For this review, take the finished solid that the model builds, in its own axes (mm). Face numbers are marked on the shaded views. A direction names the side the tool comes from. Coordinates: 2 decimals unless noted, no trailing zeros. Loops run counter-clockwise (first coordinate to the right, second up) from the corner with the lowest first, then second, coordinate; pieces in that order, holes last. Notation, with made-up numbers: M -19,-10 L -9,-10 A7 ccw -9,-1 Z; hole C -13,78.5 d4. An arc over 180 degrees is marked long. Put each result on its own line as item: value.
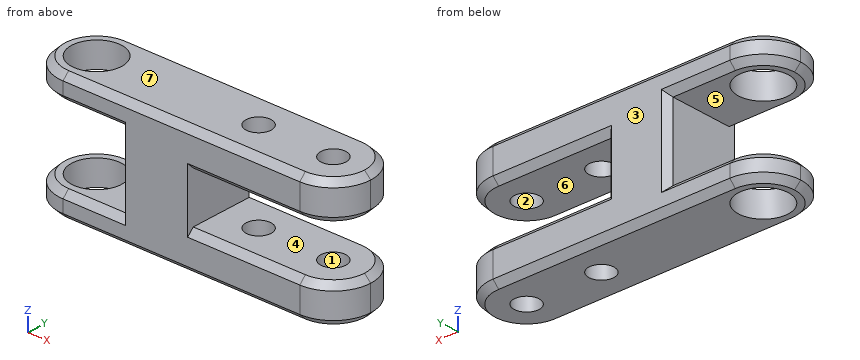
```python
from build123d import *

# Parameters (mm, degrees)
BOSS_EXTRUDE1_DEPTH       = 6
FILLET1_R                 = 3
F_4_0MM_DOWEL_HOLE1_D     = 4
F_4_0MM_DOWEL_HOLE1_DEPTH = 10
F_4_0MM_DOWEL_HOLE1_TIP   = 1.201721238
F_2_0MM_DOWEL_HOLE1_D     = 2
F_2_0MM_DOWEL_HOLE1_DEPTH = 10
F_2_0MM_DOWEL_HOLE1_TIP   = 0.600860619
CHAMFER1_SIZE             = 0.5


with BuildPart() as part:
    # Sketch2 → Boss-Extrude1 (new body)
    with BuildSketch(Plane(origin=(0, 0, 0), x_dir=(1, 0, 0), z_dir=(0, 1, 0))):
        Polygon((0, 3), (0, 5), (25, 5), (25, 2), (13, 2), (13, -2), (25, -2), (25, -5), (0, -5), (0, -3), (8, -3), (8, 3), align=None)
    extrude(amount=BOSS_EXTRUDE1_DEPTH)

    # Fillet1
    fillet1_edges = [part.edges().sort_by_distance(p)[0] for p in [
        (25, 6, -3.5),
        (25, 0, -3.5),
        (25, 0, 3.5),
        (25, 6, 3.5),
        (0, 6, 4),
        (0, 0, 4),
        (0, 0, -4),
        (0, 6, -4),
    ]]
    fillet(fillet1_edges, radius=FILLET1_R - 0.0001)  # a hair under: the kernel refuses the full size

    # Ø4.0mm Dowel Hole1
    with Locations(Plane.XY.offset(5)):
        with Locations((3, 3)):
            Hole(F_4_0MM_DOWEL_HOLE1_D / 2, depth=F_4_0MM_DOWEL_HOLE1_DEPTH)
            with Locations((0, 0, -(F_4_0MM_DOWEL_HOLE1_DEPTH + F_4_0MM_DOWEL_HOLE1_TIP / 2))):  # 118° drill point
                Cone(0, F_4_0MM_DOWEL_HOLE1_D / 2, F_4_0MM_DOWEL_HOLE1_TIP, mode=Mode.SUBTRACT)

    # Ø2.0mm Dowel Hole1
    with Locations(Plane(origin=(16, 3, 5), x_dir=(1, 0, 0), z_dir=(0, 0, 1))):
        with Locations((0, 0), (6, 0)):
            Hole(F_2_0MM_DOWEL_HOLE1_D / 2, depth=F_2_0MM_DOWEL_HOLE1_DEPTH)
            with Locations((0, 0, -(F_2_0MM_DOWEL_HOLE1_DEPTH + F_2_0MM_DOWEL_HOLE1_TIP / 2))):  # 118° drill point
                Cone(0, F_2_0MM_DOWEL_HOLE1_D / 2, F_2_0MM_DOWEL_HOLE1_TIP, mode=Mode.SUBTRACT)

    # Chamfer1
    chamfer1_edges = [part.edges().sort_by_distance(p)[0] for p in [
        (5.49995, 6, 3),
        (17.50005, 0, -2),
        (5.49995, 0, 3),
        (13, 6, 0),
        (5.49995, 6, -3),
        (12.5, 6, 5),
        (17.50005, 6, 2),
        (17.50005, 6, -2),
        (12.5, 6, -5),
        (12.5, 0, -5),
        (0.878650367, 5.121349633, -5),
        (0.878650367, 0.878650367, -5),
        (24.121349633, 0.878650367, -5),
        (24.121349633, 5.121349633, -5),
        (24.121349633, 0.878650367, -2),
        (24.121349633, 5.121349633, -2),
        (5.49995, 0, -3),
        (17.50005, 0, 2),
        (12.5, 0, 5),
        (24.121349633, 5.121349633, 2),
        (24.121349633, 0.878650367, 2),
        (0.878650367, 0.878650367, 5),
        (0.878650367, 5.121349633, 5),
        (24.121349633, 5.121349633, 5),
        (24.121349633, 0.878650367, 5),
        (0.878650367, 0.878650367, 3),
        (0.878650367, 5.121349633, 3),
        (0.878650367, 5.121349633, -3),
        (0.878650367, 0.878650367, -3),
        (8, 6, 0),
    ]]
    chamfer(chamfer1_edges, length=CHAMFER1_SIZE)


solid = part.part
```
(1) For pin 1 (3 mm diameter, centred on y = 5, z = 1, fed in from -X); pin 2 (1.5 mm diameter, centred on y = 2, z = 0, fed in from +X), all flat-tipped, find the tip position at first contact; note any pin that passes through.
Determined:
pin 1: stops at x = 8
pin 2: stops at x = 13
(2) Add section B-B (x = 18.5). Write out the cut boundary in (y, z), plus the area to 3 significant figures.
Determined:
outline: M 0,-4.5 L 0.5,-5 L 5.5,-5 L 6,-4.5 L 6,-2.5 L 5.5,-2 L 0.5,-2 L 0,-2.5 Z; M 0,2.5 L 0.5,2 L 5.5,2 L 6,2.5 L 6,4.5 L 5.5,5 L 0.5,5 L 0,4.5 Z
area: 35.0 mm^2
(3) Add section A-A (x = 16). Write out the cut boundary in (y, z).
Determined:
outline: M 0,-4.5 L 0.5,-5 L 2,-5 L 2,-2 L 0.5,-2 L 0,-2.5 Z; M 0,2.5 L 0.5,2 L 2,2 L 2,5 L 0.5,5 L 0,4.5 Z; M 4,-5 L 5.5,-5 L 6,-4.5 L 6,-2.5 L 5.5,-2 L 4,-2 Z; M 4,2 L 5.5,2 L 6,2.5 L 6,4.5 L 5.5,5 L 4,5 Z
(4) Add section C-C (z = 1). Write out the cut boundary in (x, y), plus the area to 4 significant figures.
Determined:
outline: M 8,0 L 13,0 L 13,5.5 L 12.5,6 L 8.5,6 L 8,5.5 Z
area: 29.75 mm^2
(5) Add section D-D (x = 6.25). Write out the cut boundary in (y, z), plus the area to 3 significant figures.
Determined:
outline: M 0,-4.5 L 0.5,-5 L 5.5,-5 L 6,-4.5 L 6,-3.5 L 5.5,-3 L 0.5,-3 L 0,-3.5 Z; M 0,3.5 L 0.5,3 L 5.5,3 L 6,3.5 L 6,4.5 L 5.5,5 L 0.5,5 L 0,4.5 Z
area: 23.0 mm^2
(6) Wall thickness on line 1 along Y through (x, z) = (3, -3.9); line 2 along Z through (x, y) = (18.75, 0.75); line 3 along X through (y, z) = (3, -2.8): over which ranges is each line inside the solid? List them lowest first. Write a range as [from, to].
Determined:
line 1: y = [0, 1], [5, 6]
line 2: z = [-5, -2], [2, 5]
line 3: x = [8, 15], [17, 21], [23, 25]
(7) Draft analysis for pull direction Y (two halves, no side actions). For the marked faces 1, 2, 3 and 4, state which applies: +Y half, -Y half, draft (parallel to the pull), parting line (faces both ways), or undercut.
Determined:
face 1: undercut
face 2: undercut
face 3: +Y half
face 4: draft
(8) Tool access review of the marked faces 5, 6 and 7: name each direction out of +Z, -Z, +X, -X, +Y, -Y from which nothing blocks a thin tool from reaching the whole face with its end or side.
Determined:
face 5: -X, +Y, -Y
face 6: +X, +Y, -Y
face 7: +Z, +X, -X, +Y, -Y
